Could you check a few things on this model? Use its own coordinates, in mm. A direction names the side the tool comes from. Give positions to 0.01 mm unless a question says otherwise; leave off trailing zeros. Loops run counter-clockwise (first coordinate to the right, second up) from the corner with the lowest first, then second, coordinate; pieces in that order, holes last. Notation, with made-up numbers: M 28.5,76.5 L 82.5,76.5 A21 ccw 82.5,86.5 Z; hole C 83,63.25 d8. An arc over 180 degrees is marked long. Use a Markdown table: item, result. Add a question column.
1) Will these pins go through, and if not, where does the flat tip stop? pin 1 Ø2 at (x, z) = (165, 60.5) entering from +Y; pin 2 Ø5 at (x, y) = (162, 46.5) entering from -Z; pin 3 Ø23 at (x, y) = (47.5, 48.5) entering from +Z.
2) Suppose I cut it at D-D on z = -116.5. List the corners of the cut face in (x, y) for me (3 decimals), and give its area (3 significant figures).
3) Suppose I cut it at C-C on x = 5. List the corners of the cut face in (y, z) for me.
4) Suppose I cut it at B-B on z = 188. List the corners of the cut face in (x, y) for me (3 decimals), and give its area (3 significant figures).
5) If I drill on line 1 along X through (y, z) = (44, 187) (3 decimals); line 2 along Z through (x, y) = (168, 41.5); line 3 along X through (y, z) = (75.5, 54.5) (3 decimals), over which ranges is the centre line in solid material (lowest first)? Write a range as [from, to].
6) Which directions (+Z, -Z, +X, -X, +Y, -Y) give clear straight access to the entire face, cutting with the end or side of a thin tool? Please do faces 4 (the flat face through (-3, 39, 177.8)), 5 (the flat face through (3, 41, -171.45)), 6 (the flat face through (231.775, 39, -216)).
7) We'd pull the mould along Z, two halves only. Please class faces 1 (the flat face through (-6, 2.54, -3)), 2 (the flat face through (-231.775, 39, -215)), 3 (the flat face through (319, 39, -254)): +Z half, -Z half, draft (parallel to the pull), parting line (faces both ways), or undercut.
8) Suppose I cut it at A-A on y = 63. List the corners of the cut face in (x, z) for me (3 decimals).
```python
from build123d import *

# Parameters (mm, degrees)
SKETCH1_W           = 806.45
SKETCH1_H           = 508
BOSS_EXTRUDE1_DEPTH = 2.54
SKETCH2_W           = 463.55
SKETCH2_H           = 76.2
CUT_EXTRUDE1_DEPTH  = 2.54
BOSS_EXTRUDE2_DEPTH = 77.47


with BuildPart() as part:
    # Sketch1 → Boss-Extrude1 (new body)
    with BuildSketch(Plane(origin=(0, 0, 0), x_dir=(1, 0, 0), z_dir=(0, 1, 0))):
        Rectangle(SKETCH1_W, SKETCH1_H)
    extrude(amount=BOSS_EXTRUDE1_DEPTH)

    # Sketch2 → Cut-Extrude1 (cut)
    with BuildSketch(Plane(origin=(0, 2.54, 0), x_dir=(1, 0, 0), z_dir=(0, 1, 0))):
        with Locations((0, -215.9)):
            Rectangle(SKETCH2_W, SKETCH2_H)
        with Locations((0, 215.9)):
            Rectangle(SKETCH2_W, SKETCH2_H)
    extrude(amount=-CUT_EXTRUDE1_DEPTH, mode=Mode.SUBTRACT)

    # Sketch3 → Boss-Extrude2 (add)
    with BuildSketch(Plane(origin=(0, 2.54, 0), x_dir=(1, 0, 0), z_dir=(0, 1, 0))):
        Polygon((-231.775, -254), (-231.775, -177.8), (231.775, -177.8), (231.775, -254), (403.225, -254), (403.225, 254), (231.775, 254), (231.775, 177.8), (-231.775, 177.8), (-231.775, 254), (-403.225, 254), (-403.225, -254), align=None)
        Polygon((238.125, 171.45), (-238.125, 171.45), (-238.125, 247.65), (-396.875, 247.65), (-396.875, -247.65), (-238.125, -247.65), (-238.125, -171.45), (238.125, -171.45), (238.125, -247.65), (396.875, -247.65), (396.875, 247.65), (238.125, 247.65), align=None, mode=Mode.SUBTRACT)
    extrude(amount=BOSS_EXTRUDE2_DEPTH)


solid = part.part
```
Answer block:
| question | item | result |
|---|---|---|
| 1 | pin 1 | stops at y = 2.54 |
| 1 | pin 2 | stops at z = -177.8 |
| 1 | pin 3 | stops at z = 177.8 |
| 2 | outline | M -403.225,0 L 403.225,0 L 403.225,80.01 L 396.875,80.01 L 396.875,2.54 L -396.875,2.54 L -396.875,80.01 L -403.225,80.01 Z |
| 2 | area | 3,030 mm^2 |
| 3 | outline | M 0,-177.8 L 80.01,-177.8 L 80.01,-171.45 L 2.54,-171.45 L 2.54,171.45 L 80.01,171.45 L 80.01,177.8 L 0,177.8 Z |
| 4 | outline | M -403.225,0 L -231.775,0 L -231.775,80.01 L -238.125,80.01 L -238.125,2.54 L -396.875,2.54 L -396.875,80.01 L -403.225,80.01 Z; M 231.775,0 L 403.225,0 L 403.225,80.01 L 396.875,80.01 L 396.875,2.54 L 238.125,2.54 L 238.125,80.01 L 231.775,80.01 Z |
| 4 | area | 2,840 mm^2 |
| 5 | line 1 | x = [-403.225, -396.875], [-238.125, -231.775], [231.775, 238.125], [396.875, 403.225] |
| 5 | line 2 | z = [-177.8, -171.45], [171.45, 177.8] |
| 5 | line 3 | x = [-403.225, -396.875], [396.875, 403.225] |
| 6 | face 4 | +Z, +Y, -Y |
| 6 | face 5 | +Y |
| 6 | face 6 | -Z, +Y, -Y |
| 7 | face 1 | undercut |
| 7 | face 2 | draft |
| 7 | face 3 | -Z half |
| 8 | outline | M -403.225,-254 L -231.775,-254 L -231.775,-177.8 L 231.775,-177.8 L 231.775,-254 L 403.225,-254 L 403.225,254 L 231.775,254 L 231.775,177.8 L -231.775,177.8 L -231.775,254 L -403.225,254 Z; hole M -396.875,-247.65 L -238.125,-247.65 L -238.125,-171.45 L 238.125,-171.45 L 238.125,-247.65 L 396.875,-247.65 L 396.875,247.65 L 238.125,247.65 L 238.125,171.45 L -238.125,171.45 L -238.125,247.65 L -396.875,247.65 Z |
